```python
from build123d import *

# Parameters (mm, degrees)
SKIZZE1_W                       = 200
SKIZZE1_H                       = 50
AUFSATZ_LINEAR_AUSTRAGEN1_DEPTH = 4
FASE1_SIZE                      = 25
AUFSATZ_LINEAR_AUSTRAGEN2_DEPTH = 10
SKIZZE3_W                       = 15.35533906
SKIZZE3_H                       = 10
SCHNITT_LINEAR_AUSTRAGEN1_DEPTH = 10
SKIZZE4_W                       = 15.35533906
SKIZZE4_H                       = 10
SCHNITT_LINEAR_AUSTRAGEN2_DEPTH = 10
SKIZZE5_W                       = 150
SKIZZE5_H                       = 12
AUFSATZ_LINEAR_AUSTRAGEN3_DEPTH = 5
AUFSATZ_LINEAR_AUSTRAGEN4_DEPTH = 10
AUFSATZ_LINEAR_AUSTRAGEN5_DEPTH = 10
SKIZZE11_R                      = 1.65
SKIZZE11_W                      = 2.95533906
SKIZZE11_H                      = 4
SCHNITT_LINEAR_AUSTRAGEN7_DEPTH = 10
SKIZZE12_R                      = 2.2
SCHNITT_LINEAR_AUSTRAGEN8_DEPTH = 10
AUFSATZ_LINEAR_AUSTRAGEN6_DEPTH = 10
SKIZZE8_R                       = 1.65
SKIZZE8_W                       = 3.016289267
SKIZZE8_H                       = 4
SCHNITT_LINEAR_AUSTRAGEN9_DEPTH = 10
KREISMUSTER1_START              = 56.301499416
KREISMUSTER1_OUTLINE_R          = 1.65
KREISMUSTER1_DEPTH              = 0.969560509
KREISMUSTER1_START_2            = 64.310678119
KREISMUSTER1_2_OUTLINE_W        = 0.949011964
KREISMUSTER1_2_OUTLINE_H        = 10
KREISMUSTER1_2_OUTLINE_R        = 1.65
KREISMUSTER1_2_OUTLINE_W_2      = 1.050988037
KREISMUSTER1_2_OUTLINE_W_3      = 2.955339059
KREISMUSTER1_2_OUTLINE_H_2      = 4
KREISMUSTER1_2_DEPTH            = 1.990821297
KREISMUSTER1_START_3            = 66.301499416
KREISMUSTER1_3_OUTLINE_R        = 1.65
KREISMUSTER1_3_OUTLINE_W        = 2.955339059
KREISMUSTER1_3_OUTLINE_H        = 4
KREISMUSTER1_3_DEPTH            = 0.009178703
KREISMUSTER1_START_4            = 64.242319383
KREISMUSTER1_4_OUTLINE_R        = 1.65
KREISMUSTER1_4_DEPTH            = 6.4
AUFSATZ_LINEAR_AUSTRAGEN7_DEPTH = 10
KREISMUSTER2_COUNT              = 2


# Read off the part's stored shape, not the designer's step: Kreismuster1
with BuildPart() as part:
    # Skizze1 → Aufsatz-Linear austragen1 (new body)
    with BuildSketch(Plane(origin=(0, 0, 0), x_dir=(1, 0, 0), z_dir=(0, 1, 0))):
        Rectangle(SKIZZE1_W, SKIZZE1_H)
    extrude(amount=AUFSATZ_LINEAR_AUSTRAGEN1_DEPTH)

    # Fase1
    fase1_edges = [part.edges().sort_by_distance(p)[0] for p in [
        (-100, 2, -25),
        (-100, 2, 25),
        (100, 2, -25),
        (100, 2, 25),
    ]]
    chamfer(fase1_edges, length=FASE1_SIZE - 0.0001)  # a hair under: the kernel refuses the full size

    # Skizze2 → Aufsatz-Linear austragen2 (add)
    with BuildSketch(Plane(origin=(0, 4, 0), x_dir=(1, 0, 0), z_dir=(0, 1, 0))):
        Polygon((-73.177460326, 20.6), (-93.777460326, 0), (-73.277460326, -20.5), (73.277460326, -20.5), (93.777460326, 0), (73.177460326, 20.6), align=None)
        Polygon((90.949033201, 0), (72.349033201, 18.6), (-72.349033201, 18.6), (-90.949033201, 0), (-72.449033201, -18.5), (72.449033201, -18.5), align=None, mode=Mode.SUBTRACT)
    extrude(amount=AUFSATZ_LINEAR_AUSTRAGEN2_DEPTH)

    # Skizze3 → Schnitt-Linear austragen1 (cut)
    with BuildSketch(Plane(origin=(-46.888730163, 0, 46.888730163), x_dir=(0.7071067811865476, 0, 0.7071067811865476), z_dir=(-0.7071067811865476, 0, 0.7071067811865476))):
        with Locations((-53.033008589, 9)):
            Rectangle(SKIZZE3_W, SKIZZE3_H)
    extrude(amount=-SCHNITT_LINEAR_AUSTRAGEN1_DEPTH, mode=Mode.SUBTRACT)

    # Skizze4 → Schnitt-Linear austragen2 (cut)
    with BuildSketch(Plane(origin=(46.888730163, 0, 46.888730163), x_dir=(0.7071067811865475, 0, -0.7071067811865477), z_dir=(0.7071067811865477, 0, 0.7071067811865475))):
        with Locations((53.033008589, 9)):
            Rectangle(SKIZZE4_W, SKIZZE4_H)
    extrude(amount=-SCHNITT_LINEAR_AUSTRAGEN2_DEPTH, mode=Mode.SUBTRACT)

    # Skizze5 → Aufsatz-Linear austragen3 (add)
    with BuildSketch(Plane(origin=(0, 4, 0), x_dir=(1, 0, 0), z_dir=(0, 1, 0))):
        with Locations((-0.006490323, 0)):
            Rectangle(SKIZZE5_W, SKIZZE5_H)
    extrude(amount=AUFSATZ_LINEAR_AUSTRAGEN3_DEPTH)

    # Skizze6 → Aufsatz-Linear austragen4 (add)
    with BuildSketch(Plane(origin=(0, 4, 0), x_dir=(1, 0, 0), z_dir=(0, 1, 0))):
        Polygon((87.696342007, -3.252691193), (78.252691193, -12.696342007), (82.735076288, -17.264923712), (92.221825407, -7.778174593), align=None)
    aufsatz_linear_austragen4 = extrude(amount=AUFSATZ_LINEAR_AUSTRAGEN4_DEPTH)

    # Skizze10 → Aufsatz-Linear austragen5 (add)
    with BuildSketch(Plane(origin=(0, 4, 0), x_dir=(1, 0, 0), z_dir=(0, 1, 0))):
        Polygon((-87.696342007, -3.252691193), (-78.252691193, -12.696342007), (-82.778174593, -17.221825407), (-92.221825407, -7.778174593), align=None)
    extrude(amount=AUFSATZ_LINEAR_AUSTRAGEN5_DEPTH)

    # Skizze11 → Schnitt-Linear austragen7 (cut)
    with BuildSketch(Plane(origin=(-50, 0, 50), x_dir=(0.7071067811865465, 0, 0.7071067811865488), z_dir=(-0.7071067811865488, 0, 0.7071067811865465))):
        with Locations((-56.710678119, 9)):
            Circle(SKIZZE11_R)
        with Locations((-49.355339059, 9)):
            Circle(SKIZZE11_R)
        with Locations((-53.033008589, 6)):
            Rectangle(SKIZZE11_W, SKIZZE11_H)
    extrude(amount=-SCHNITT_LINEAR_AUSTRAGEN7_DEPTH, mode=Mode.SUBTRACT)

    # Skizze12 → Schnitt-Linear austragen8 (cut)
    with BuildSketch(Plane(origin=(0, 4, 0), x_dir=(1, 0, 0), z_dir=(0, 1, 0))):
        with Locations(Location((0, 12.5, 0), (0, 0, 270))):
            Circle(SKIZZE12_R)
        with Locations(Location((0, -12.5, 0), (0, 0, 270))):
            Circle(SKIZZE12_R)
    extrude(amount=-SCHNITT_LINEAR_AUSTRAGEN8_DEPTH, mode=Mode.SUBTRACT)

    # Skizze13 → Aufsatz-Linear austragen6 (add)
    with BuildSketch(Plane(origin=(0, 4, 0), x_dir=(1, 0, 0), z_dir=(0, 1, 0))):
        Polygon((89.817662351, -3.959797975), (88.403448789, -2.545584412), (87.69285367, -3.256179531), (89.107067232, -4.670393094), align=None)
        Polygon((-89.817662351, -3.959797975), (-88.403448789, -2.545584412), (-87.689553601, -3.2594796), (-89.103767163, -4.673693162), align=None)
        Polygon((78.959797975, -14.817662351), (77.545584412, -13.403448789), (78.257117259, -12.691915942), (79.671330821, -14.106129505), align=None)
        Polygon((-78.959797975, -14.817662351), (-77.545584412, -13.403448789), (-78.262212477, -12.686820723), (-79.67642604, -14.101034286), align=None)
    aufsatz_linear_austragen6 = extrude(amount=AUFSATZ_LINEAR_AUSTRAGEN6_DEPTH)

    # Skizze8 → Schnitt-Linear austragen9 (cut)
    with BuildSketch(Plane(origin=(50, 0, 50), x_dir=(0.7071067811865488, 0, -0.7071067811865465), z_dir=(0.7071067811865465, 0, 0.7071067811865488))):
        with Locations((49.294388852, 9)):
            Circle(SKIZZE8_R)
        with Locations((56.710678119, 9)):
            Circle(SKIZZE8_R)
        with Locations((53.002533486, 6)):
            Rectangle(SKIZZE8_W, SKIZZE8_H)
    schnitt_linear_austragen9 = extrude(amount=-SCHNITT_LINEAR_AUSTRAGEN9_DEPTH, mode=Mode.SUBTRACT)

    # Kreismuster1 outline → Kreismuster1 (cut)
    with BuildSketch(Plane(origin=(0, 0, 0), x_dir=(0.707106781186546, 0, 0.707106781186549), z_dir=(0.707106781186549, 0, -0.707106781186546)).offset(KREISMUSTER1_START)):
        Polygon((46.29517232, -9), (46.29517232, -14), (59.650511379, -14), (59.650511379, -4), (54.450511379, -4), (54.450511379, -8), (51.49517232, -8), (51.49517232, -4), (46.29517232, -4), align=None)
        with BuildLine():
            Line((47.64517232, -9), (50.94517232, -9))
            ThreePointArc((50.94517232, -9), (49.29517232, -10.65), (47.64517232, -9))
        make_face(mode=Mode.SUBTRACT)
        with Locations((56.650511379, -9)):
            Circle(KREISMUSTER1_OUTLINE_R, mode=Mode.SUBTRACT)
    extrude(amount=KREISMUSTER1_DEPTH, mode=Mode.SUBTRACT)

    # Kreismuster1 2 outline → Kreismuster1 2 (cut)
    with BuildSketch(Plane(origin=(0, 0, 0), x_dir=(0.707106781186546, 0, 0.707106781186549), z_dir=(0.707106781186549, 0, -0.707106781186546)).offset(KREISMUSTER1_START_2)):
        with Locations((45.820666338, -9)):
            Rectangle(KREISMUSTER1_2_OUTLINE_W, KREISMUSTER1_2_OUTLINE_H)
        with Locations((56.650511379, -9)):
            Circle(KREISMUSTER1_2_OUTLINE_R)
        with Locations((49.29517232, -9)):
            Circle(KREISMUSTER1_2_OUTLINE_R)
        with Locations((60.176005398, -9)):
            Rectangle(KREISMUSTER1_2_OUTLINE_W_2, KREISMUSTER1_2_OUTLINE_H)
        with Locations((52.972841849, -6)):
            Rectangle(KREISMUSTER1_2_OUTLINE_W_3, KREISMUSTER1_2_OUTLINE_H_2)
    extrude(amount=KREISMUSTER1_2_DEPTH, mode=Mode.SUBTRACT)

    # Kreismuster1 3 outline → Kreismuster1 3 (cut)
    with BuildSketch(Plane(origin=(0, 0, 0), x_dir=(0.707106781186546, 0, 0.707106781186549), z_dir=(0.707106781186549, 0, -0.707106781186546)).offset(KREISMUSTER1_START_3)):
        with Locations((56.650511379, -9)):
            Circle(KREISMUSTER1_3_OUTLINE_R)
        with Locations((49.29517232, -9)):
            Circle(KREISMUSTER1_3_OUTLINE_R)
        with Locations((52.972841849, -6)):
            Rectangle(KREISMUSTER1_3_OUTLINE_W, KREISMUSTER1_3_OUTLINE_H)
    extrude(amount=KREISMUSTER1_3_DEPTH, mode=Mode.SUBTRACT)

    # Kreismuster1 4 outline → Kreismuster1 4 (add)
    with BuildSketch(Plane(origin=(0, 0, 0), x_dir=(0.707106781186546, 0, 0.707106781186549), z_dir=(0.707106781186549, 0, -0.707106781186546)).offset(KREISMUSTER1_START_4)):
        Polygon((46.29517232, -9), (46.29517232, -14), (59.650511379, -14), (59.650511379, -4), (54.450511379, -4), (54.450511379, -8), (51.49517232, -8), (51.49517232, -4), (46.29517232, -4), align=None)
        with BuildLine():
            ThreePointArc((50.94517232, -9), (49.29517232, -10.65), (47.64517232, -9))
            ThreePointArc((47.64517232, -9), (49.29517232, -7.35), (50.94517232, -9))
        make_face(mode=Mode.SUBTRACT)
        with Locations((56.650511379, -9)):
            Circle(KREISMUSTER1_4_OUTLINE_R, mode=Mode.SUBTRACT)
    extrude(amount=KREISMUSTER1_4_DEPTH)

    # Skizze14 → Aufsatz-Linear austragen7 (add)
    with BuildSketch(Plane(origin=(0, 4, 0), x_dir=(1, 0, 0), z_dir=(0, 1, 0))):
        Polygon((88.396958465, 2.552074735), (89.804681705, 3.959797975), (89.061520937, 4.702958742), (87.653797698, 3.295235503), align=None)
        Polygon((77.539094089, 13.409939112), (78.946817328, 14.817662351), (79.612825848, 14.151653831), (78.205102609, 12.743930592), align=None)
    extrude(amount=AUFSATZ_LINEAR_AUSTRAGEN7_DEPTH)

    # Kreismuster2: Aufsatz-Linear austragen4, Aufsatz-Linear austragen6, Schnitt-Linear austragen9 ×2 about axis
    kreismuster2_axis = Axis((-0.045440618, 0, 0.002896308), (0, 1, 0))
    add([aufsatz_linear_austragen4.rotate(kreismuster2_axis, i * 360 / KREISMUSTER2_COUNT) for i in range(1, KREISMUSTER2_COUNT)])
    add([aufsatz_linear_austragen6.rotate(kreismuster2_axis, i * 360 / KREISMUSTER2_COUNT) for i in range(1, KREISMUSTER2_COUNT)])
    add([schnitt_linear_austragen9.rotate(kreismuster2_axis, i * 360 / KREISMUSTER2_COUNT) for i in range(1, KREISMUSTER2_COUNT)], mode=Mode.SUBTRACT)


solid = part.part
```
Geometry: final body of the model. Coordinates: model frame, mm. A direction names the side the tool comes from. Coordinates: 2 decimals unless noted, no trailing zeros. Order: outer loops, then holes, each group sorted by start corner. A loop starts at its lowest first (then second) coordinate and runs counter-clockwise, first axis right, second up. Notation, with made-up numbers: (4, -33) -> (25, -33) arc R28 cw to (25, 1) -> close; hole circle Ø11 at (40, 8.25). An arc over 180 degrees is marked (long way). Write each question's results on one line, items separated by ' | '. Start each with the question number.
1) Cut plane B-B, the plane y = 1.75. State how many separate pieces and enclosed holes the cut face has, and give its area (3 significant figures).
2) First-contact query: pin 1 (5 mm diameter, centred on y = 9.5, z = 9.5, fed in from +X); pin 2 (2.5 mm diameter, centred on y = 6.5, z = 0.5, fed in from +X); pin 3 (8 mm diameter, centred on y = 4.5, z = -19.5, fed in from -X); pin 4 (2.5 mm diameter, centred on x = 0, z = -12.5, fed in from +Y). Flat tips, straight axial feed; report the tip coordinate or a pass-through.
3) Material intervals for line 1 along Z through (x, y) = (-30, 13.25); line 2 along Z through (x, y) = (86, 7.75); line 3 along X through (y, z) = (5.25, 3), sorted ascending.
4) Mould query, pull axis Z, two halves, no side actions, for faces 1 (the flat face through (-1, 9, 18.5)), 2 (the flat face through (-1, 0, 0)), 3 (the flat face through (-87, 2, -13)). Classes: released by +Z, released by -Z, zero draft, split by the parting line, or undercut.
5) Cut plane C-C, the plane x = 37.5. Output: boundary loops of the cut face in (y, z).
6) Cut plane A-A, the plane x = 0. Output: boundary loops of the cut face in (y, z), and give its area (3 significant figures).
7) Set-up query: faces 4 (the flat face through (-76.52, 8.93, 17.26)), 5 (the flat face through (84.07, 6.028, -11.245)), 6 (the flat face through (-1, 9, 20.5)), 7 (the flat face through (91.46, 8.93, -2.32)). Return all of +Z, -Z, +X, -X, +Y, -Y with unobstructed straight access to the full face (end or side cutting, diameter ignored); none if empty.
Checks:
1) separate pieces: 1 | enclosed holes: 2 | area: 8,720 mm^2
2) pin 1: x = 92.22 | pin 2: x = 93.78 | pin 3: x = -84.59 | pin 4: through
3) line 1: -20.6 to -18.6, 18.5 to 20.5 | line 2: -13.9 to -13.17, -9 to -7.41, 7.32 to 8.91, 13.18 to 14 | line 3: -90.78 to -87.95, -75.01 to 74.99, 87.95 to 90.78
4) face 1: undercut | face 2: zero draft | face 3: released by -Z
5) outline: (0, -25) -> (4, -25) -> (4, -20.6) -> (14, -20.6) -> (14, -18.6) -> (4, -18.6) -> (4, -6) -> (9, -6) -> (9, 6) -> (4, 6) -> (4, 18.5) -> (14, 18.5) -> (14, 20.5) -> (4, 20.5) -> (4, 25) -> (0, 25) -> close
6) outline: (0, -25) -> (4, -25) -> (4, -20.6) -> (14, -20.6) -> (14, -18.6) -> (4, -18.6) -> (4, -14.7) -> (0, -14.7) -> close; (0, -10.3) -> (4, -10.3) -> (4, -6) -> (9, -6) -> (9, 6) -> (4, 6) -> (4, 10.3) -> (0, 10.3) -> close; (0, 14.7) -> (4, 14.7) -> (4, 18.5) -> (14, 18.5) -> (14, 20.5) -> (4, 20.5) -> (4, 25) -> (0, 25) -> close | area: 265 mm^2
7) face 4: +Z, +Y | face 5: none | face 6: +Z, +X, -X, +Y | face 7: +X, +Y
